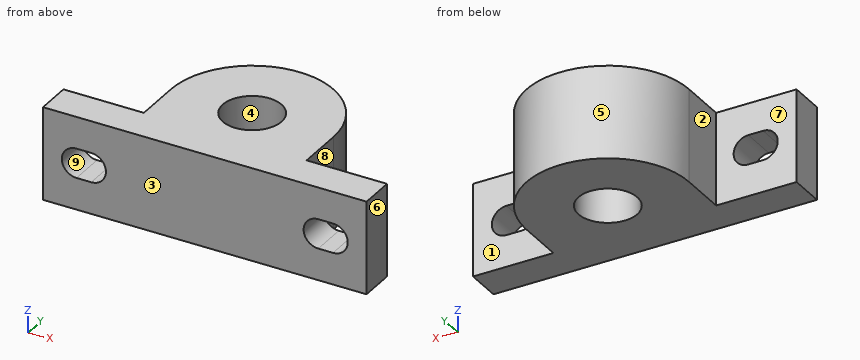
from build123d import *

# Parameters (mm, degrees)
SKETCH2_R                      = 12.7
BOSS_EXTRUDE1_DEPTH            = 40.1066
F_1_2_0_5_DIAMETER_SLOT1_DEPTH = 15.24


# Read off the part's stored shape, not the designer's step: 1/2 (0.5) Diameter Slot1
with BuildPart() as part:
    # Sketch2 → Boss-Extrude1 (new body)
    with BuildSketch(Plane.XY):
        with BuildLine():
            Line((69.85, 0), (-69.85, 0))
            Line((-69.85, 0), (-69.85, 15.24))
            Line((-69.85, 15.24), (-35.1282, 15.24))
            Line((-35.1282, 15.24), (-35.1282, 35.3568))
            ThreePointArc((-35.1282, 35.3568), (0, 70.485), (35.1282, 35.3568))
            Line((35.1282, 35.3568), (35.1282, 15.24))
            Line((35.1282, 15.24), (69.85, 15.24))
            Line((69.85, 15.24), (69.85, 0))
        make_face()
        with Locations((0, 35.3568)):
            Circle(SKETCH2_R, mode=Mode.SUBTRACT)
    extrude(amount=BOSS_EXTRUDE1_DEPTH)

    # 1/2 (0.5) Diameter Slot1 outline → 1/2 (0.5) Diameter Slot1 (cut)
    with BuildSketch(Plane(origin=(0, 0, 0), x_dir=(1, 0, 0), z_dir=(0, 1, 0))):
        with BuildLine():
            Line((-55.372, -26.4033), (-49.022, -26.4033))
            ThreePointArc((-49.022, -26.4033), (-42.672, -20.0533), (-49.022, -13.7033))
            Line((-49.022, -13.7033), (-55.372, -13.7033))
            ThreePointArc((-55.372, -13.7033), (-61.722, -20.0533), (-55.372, -26.4033))
        make_face()
        with BuildLine():
            ThreePointArc((55.372, -26.4033), (61.722, -20.0533), (55.372, -13.7033))
            Line((55.372, -13.7033), (49.022, -13.7033))
            ThreePointArc((49.022, -13.7033), (42.672, -20.0533), (49.022, -26.4033))
            Line((49.022, -26.4033), (55.372, -26.4033))
        make_face()
    extrude(amount=F_1_2_0_5_DIAMETER_SLOT1_DEPTH, mode=Mode.SUBTRACT)


solid = part.part
The model under review builds one solid part; all positions refer to its coordinate system, in mm. Face numbers are marked on the shaded views. A direction names the side the tool comes from. Round coordinates to 2 decimals unless told otherwise and drop trailing zeros. Write each loop counter-clockwise with the first axis right and the second up, starting at its lowest first coordinate (ties: lowest second). Pieces come first, ordered by that corner, then holes. Notation, with made-up numbers: (61, 88) - (98, 88) arc R15 cw to (98, 100) - close; hole circle Ø9 at (-23, 47). An arc over 180 degrees is marked (long way). One line per item, written item: value. Start each with the question number.
1. Consider section C-C on y = 26.5. Write out the cut boundary in (x, z), and give its area (3 significant figures).
2. The part is to be moulded in two halves that separate along Y. For the marked faces 1, 2, 3 and 4, say which applies: released by +Y, released by -Y, zero draft, split by the parting line, or undercut.
3. Consider section B-B on z = 10.5. Write out the cut boundary in (x, y), and give its area (3 significant figures).
4. Machinability: for the marked faces 5, 6, 7, 8 and 9, which of the approach directions +Z, -Z, +X, -X, +Y, -Y give a long, thin tool a straight path to every point of the face, cutting with its end or side? Answer none if there is none.
5. Consider section D-D on z = 20.5. Write out the cut boundary in (x, y).
6. Consider section A-A on x = 0. Write out the cut boundary in (y, z) (3 decimals).
7. To check wall thickness, follow L1, parallel to Y at x = 0, z = 29 (3 decimals); L2, parallel to X at y = 42, z = 26.5; L3, parallel to Y at x = 51.5, z = 30. State the ranges of each line that lie inside material, in increasing order. Write a range as from..to.
8. Clearance check with flat-ended pins moving along their axes: P1, Ø6, axis at y = 24, z = 19, coming from the +X side; P2, Ø3, axis at y = 56.5, z = 14, coming from the -X side; P3, Ø10, axis at x = -29, y = 53.5, coming from the -Z side; P4, Ø6, axis at y = 29.5, z = 29, coming from the -X side. State where each tip first meets the part, or that it passes through.
Checks:
1. outline: (-35.13, 0) - (-9.1, 0) - (-9.1, 40.11) - (-35.13, 40.11) - close; (9.1, 0) - (35.13, 0) - (35.13, 40.11) - (9.1, 40.11) - close
1. area: 2,090 mm^2
2. face 1: released by +Y
2. face 2: zero draft
2. face 3: released by -Y
2. face 4: undercut
3. outline: (-69.85, 0) - (69.85, 0) - (69.85, 15.24) - (35.13, 15.24) - (35.13, 35.36) arc R35.13 ccw to (-35.13, 35.36) - (-35.13, 15.24) - (-69.85, 15.24) - close; hole circle Ø25.4 at (0, 35.36)
3. area: 4,970 mm^2
4. face 5: +Z, -Z, +Y
4. face 6: +Z, -Z, +X, +Y, -Y
4. face 7: +Z, -Z, -X, +Y
4. face 8: +Z, -Z, +X, +Y
4. face 9: +Y, -Y
5. outline: (-69.85, 0) - (-61.71, 0) - (-61.71, 15.24) - (-69.85, 15.24) - close; (-42.69, 0) - (42.69, 0) - (42.69, 15.24) - (35.13, 15.24) - (35.13, 35.36) arc R35.13 ccw to (-35.13, 35.36) - (-35.13, 15.24) - (-42.69, 15.24) - close; (61.71, 0) - (69.85, 0) - (69.85, 15.24) - (61.71, 15.24) - close; hole circle Ø25.4 at (0, 35.36)
6. outline: (0, 0) - (22.657, 0) - (22.657, 40.107) - (0, 40.107) - close; (48.057, 0) - (70.485, 0) - (70.485, 40.107) - (48.057, 40.107) - close
7. L1: y = 0..22.657, 48.057..70.485
7. L2: x = -34.49..-10.82, 10.82..34.49
7. L3: y = 0..15.24
8. P1: stops at x = 35.13
8. P2: stops at x = -29.12
8. P3: stops at z = 0
8. P4: stops at x = -35.13
